from build123d import *

# Parameters (mm, degrees)
BOSS_EXTRUDE1_DEPTH = 56.22
SKETCH2_R           = 2.5
CUT_EXTRUDE1_DEPTH  = 31.48
SKETCH4_R           = 2.5
CUT_EXTRUDE2_DEPTH  = 51


with BuildPart() as part:
    # Sketch1 → Boss-Extrude1 (new body)
    with BuildSketch(Plane.XY):
        with BuildLine():
            Line((45.33, -9.4), (45.33, -39.88))
            Line((45.33, -39.88), (51.7054, -39.88))
            Line((51.7054, -39.88), (51.7054, -23.3954))
            ThreePointArc((51.7054, -23.3954), (53.937246327, -18.007246327), (59.3254, -15.7754))
            Line((59.3254, -15.7754), (95.33, -15.7754))
            Line((95.33, -15.7754), (95.33, -9.4))
            Line((95.33, -9.4), (45.33, -9.4))
        make_face()
    extrude(amount=-BOSS_EXTRUDE1_DEPTH)

    # Sketch2 → Cut-Extrude1 (cut, through all)
    with BuildSketch(Plane(origin=(0, -9.4, 0), x_dir=(1, 0, 0), z_dir=(0, 1, 0))):
        with Locations((75.33, 12.493588432)):
            Circle(SKETCH2_R)
        with Locations((75.33, 32.493588432)):
            Circle(SKETCH2_R)
    extrude(amount=-CUT_EXTRUDE1_DEPTH, mode=Mode.SUBTRACT)

    # Sketch4 → Cut-Extrude2 (cut, through all)
    with BuildSketch(Plane.ZY.offset(-45.33)):
        with Locations((-32.598, -27.18)):
            Circle(SKETCH4_R)
    extrude(amount=-CUT_EXTRUDE2_DEPTH, mode=Mode.SUBTRACT)


solid = part.part
Design review of the part built by this model. Coordinates are the model's own, in mm. A direction names the side the tool comes from. Give positions to 0.01 mm unless a question says otherwise; leave off trailing zeros. Loops run counter-clockwise (first coordinate to the right, second up) from the corner with the lowest first, then second, coordinate; pieces in that order, holes last. Notation, with made-up numbers: M 67,-37.75 L 77,-37.75 A7 cw 77,-29.75 Z; hole C -35,77.25 d6. An arc over 180 degrees is marked long. One line per question, with ' | ' between items. Start each with the question number.
1. Add section D-D (y = -36.5). Write out the cut boundary in (x, z), plus the area to 3 significant figures.
2. Add section C-C (z = -20). Write out the cut boundary in (x, y).
3. Insertion check: P1, Ø8, axis at y = -34, z = -38, coming from the +X side; P2, Ø1.5, axis at y = -21, z = -50.5, coming from the +X side; P3, Ø6.5, axis at x = 75.33, z = -12.49, coming from the -Y side. Each pin has a flat end and moves straight along its axis. Give the tip position at first contact, or say it passes through.
4. Add section A-A (x = 75.33). Write out the cut boundary in (y, z), plus the area to 3 significant figures.
5. To check wall thickness, follow L1, parallel to Z at x = 75.33, y = -13.25; L2, parallel to Y at x = 66.5, z = -13; L3, parallel to X at y = -25, z = -19. State the ranges of each line that lie inside material, in increasing order.
6. For faces 1 (the face through (45.33, -24, -28)), 2 (the face through (51.705, -32, -28)), list the 3-axis set-ups (+Z, -Z, +X, -X, +Y, -Y) from which the entire face can be reached by the end or side of a thin tool; tool diameter is ignored.
7. The part is to be moulded in two halves that separate along X. For faces 3 (the face through (48, -39.88, -28)), 4 (the face through (72.832, -12.543, -12.604)), 5 (the face through (72.832, -12.543, -32.604)), 6 (the face through (95.33, -13, -28)), say which applies: released by +X, released by -X, zero draft, split by the parting line, or undercut.
8. Add section B-B (y = -27.18). Write out the cut boundary in (x, z), plus the area to 3 significant figures.
Worked out:
1) outline: M 45.33,-56.22 L 51.71,-56.22 L 51.71,0 L 45.33,0 Z | area: 358 mm²
2) outline: M 45.33,-39.88 L 51.71,-39.88 L 51.71,-23.4 A7.62 cw 59.33,-15.78 L 95.33,-15.78 L 95.33,-9.4 L 45.33,-9.4 Z
3) P1: stops at x = 51.71 | P2: stops at x = 52.38 | P3: stops at y = -15.78
4) outline: M -15.78,-56.22 L -9.4,-56.22 L -9.4,-34.99 L -15.78,-34.99 Z; M -15.78,-29.99 L -9.4,-29.99 L -9.4,-14.99 L -15.78,-14.99 Z; M -15.78,-9.99 L -9.4,-9.99 L -9.4,0 L -15.78,0 Z | area: 295 mm²
5) L1: z = -56.22 to -34.99, -29.99 to -14.99, -9.99 to 0 | L2: y = -15.78 to -9.4 | L3: x = 45.33 to 51.71
6) face 1: +Z, -Z, -X, +Y, -Y | face 2: +Z, -Z, +X, -Y
7) face 3: zero draft | face 4: undercut | face 5: undercut | face 6: released by +X
8) outline: M 45.33,-56.22 L 51.71,-56.22 L 51.71,-35.1 L 45.33,-35.1 Z; M 45.33,-30.1 L 51.71,-30.1 L 51.71,0 L 45.33,0 Z | area: 327 mm²
